Read the model definition and answer for the solid it produces. Units are mm, in the model's axes. Face numbers are marked on the shaded views. A direction names the side the tool comes from. Give positions to 0.01 mm unless a question says otherwise; leave off trailing zeros. Order: outer loops, then holes, each group sorted by start corner. A loop starts at its lowest first (then second) coordinate and runs counter-clockwise, first axis right, second up. Notation, with made-up numbers: M 66,48.25 L 119,48.25 A14 cw 119,61.25 Z; hole C 63.5,31 d9. An arc over 180 degrees is marked long. One line per item, written item: value. Start each with the question number.
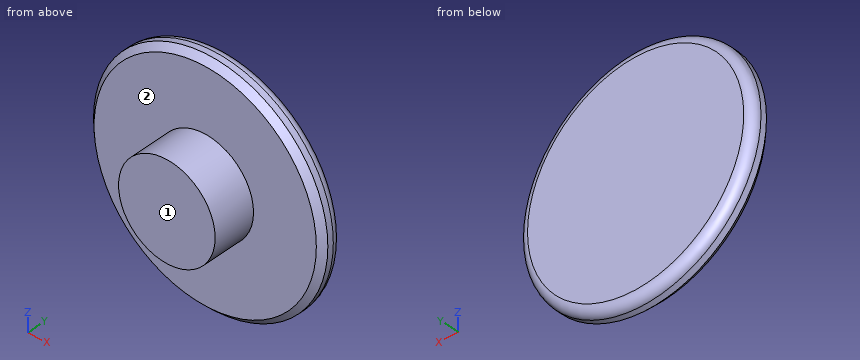
from build123d import *

# Parameters (mm, degrees)
F0_R     = 4
F1_DEPTH = 5.25
F0_R_2   = 9.7
F2_DEPTH = 1.75
F3_SIZE  = 0.5
F4_R     = 0.75


# Not quite as in the source:
# - a feature names something its author has since deleted; it is built from what else it names


with BuildPart() as f1:
    # F0 (on Front) → F1 (new body)
    with BuildSketch(Plane.XZ):
        Circle(F0_R)
    extrude(amount=F1_DEPTH)

    # F0 (on Front) → F2 (join)
    with BuildSketch(Plane.XZ):
        Circle(F0_R_2)
        Circle(F0_R, mode=Mode.SUBTRACT)
    extrude(amount=F2_DEPTH)

    # F3
    f3_edges = [f1.edges().sort_by_distance(p)[0] for p in [
        (-9.7, -1.75, 0),
    ]]
    chamfer(f3_edges, length=F3_SIZE)

    # F4
    f4_edges = [f1.edges().sort_by_distance(p)[0] for p in [
        (-9.7, 0, 0),
    ]]
    fillet(f4_edges, radius=F4_R)


solid = f1.part
Q1. Find section D-D, the plane y = -1.5. Give the vertices of the cut face in (x, z).
Q2. Find section B-B, the plane z = 0. Give the vertices of the cut face in (x, y).
Q3. A tool of negligible diameter and unlimited length cuts with its end or side. For the marked faces 1 and 2, from which of +Z, -Z, +X, -X, +Y, -Y can it reach the whole face along a straight path? Write none if from no direction.
Q4. Find section C-C, the plane y = -4.6. Give the vertices of the cut face in (x, z), then the cut area to 3 significant figures.
Q5. Consider probe 1 along Y at (x, z) = (-4, 3.75); probe 2 along Z at (x, y) = (0, -4.5); probe 3 along X at (y, z) = (-4.6, 3). Determine where each line is inside the solid, lowest interval first.
Q6. Each of these flat-tipped pins is pushed along its axis until it touches: pin 1 (1.5 mm diameter, centred on x = 7.5, z = -4.5, fed in from -Y); pin 2 (1 mm diameter, centred on y = -3, z = -4, fed in from +X); pin 3 (2 mm diameter, centred on y = -4, z = 2, fed in from -X). Where does it stop, or does it pass through?
Q7. Find section A-A, the plane x = 0. Give the vertices of the cut face in (y, z).
Evaluation:
1. outline: C 0,0 d18.9
2. outline: M -9.7,-1.25 L -9.2,-1.75 L -4,-1.75 L -4,-5.25 L 4,-5.25 L 4,-1.75 L 9.2,-1.75 L 9.7,-1.25 L 9.7,-0.75 A0.75 ccw 8.95,0 L -8.95,0 A0.75 ccw -9.7,-0.75 Z
3. face 1: +Z, -Z, +X, -X, -Y
3. face 2: -Y
4. outline: C 0,0 d8
4. area: 50.3 mm2
5. probe 1: -1.75 to 0
5. probe 2: -4 to 4
5. probe 3: -2.65 to 2.65
6. pin 1: y = -1.75
6. pin 2: x = 1.94
6. pin 3: x = -3.87
7. outline: M -5.25,-4 L -1.75,-4 L -1.75,-9.2 L -1.25,-9.7 L -0.75,-9.7 A0.75 ccw 0,-8.95 L 0,8.95 A0.75 ccw -0.75,9.7 L -1.25,9.7 L -1.75,9.2 L -1.75,4 L -5.25,4 Z
